Job drawing, mm, ordinate dimensions from the low corner. One solid piece. A direction names the side the tool comes from. Coordinates: 2 decimals unless noted, no trailing zeros. Order: outer loops, then holes, each group sorted by start corner. A loop starts at its lowest first (then second) coordinate and runs counter-clockwise, first axis right, second up. Notation, with made-up numbers: (-34.5, -22) - (-13.5, -22) arc R7 ccw to (-13.5, -17) - close; hole circle Ø9 at (44, 32). An arc over 180 degrees is marked (long way). Use one line per item in the form item = value.
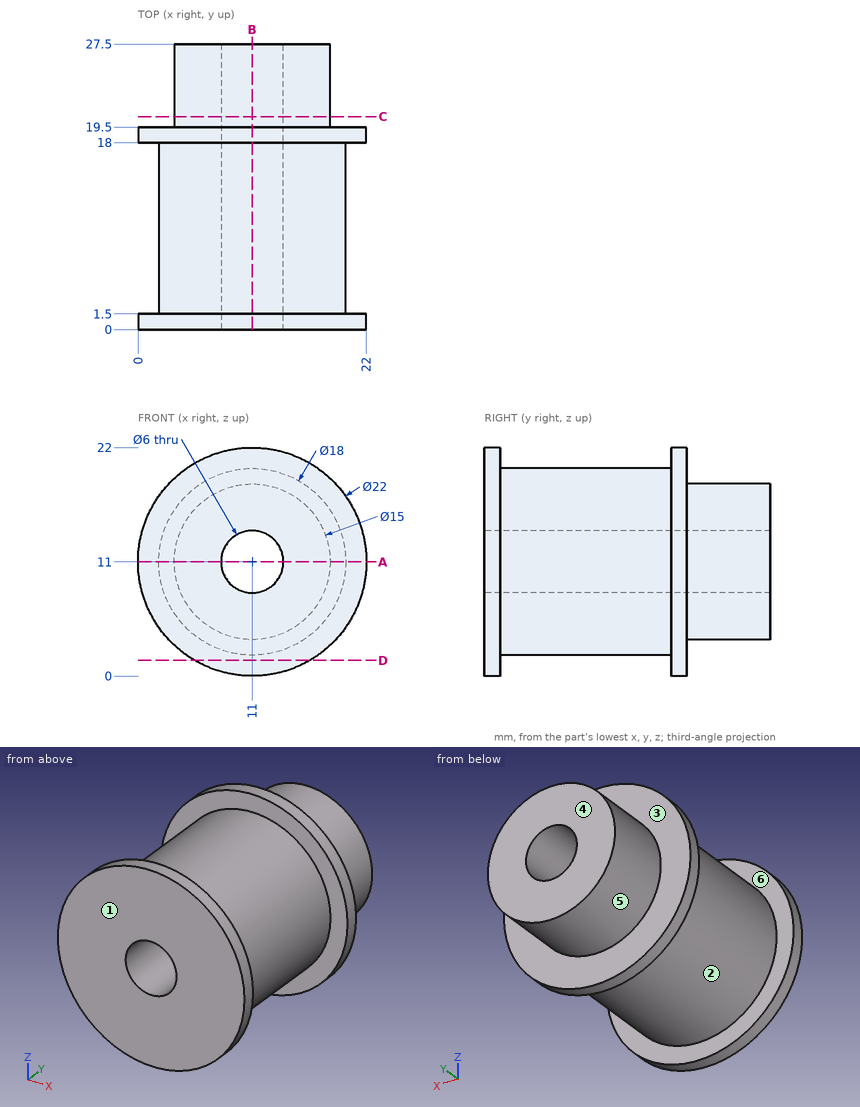
Item 1: Cut at B-B, the plane x = 11. Write the cut outline in (y, z), plus the area to 3 significant figures.
Derived:
outline = (0, 0) - (1.5, 0) - (1.5, 2) - (18, 2) - (18, 0) - (19.5, 0) - (19.5, 3.5) - (27.5, 3.5) - (27.5, 8) - (0, 8) - close; (0, 14) - (27.5, 14) - (27.5, 18.5) - (19.5, 18.5) - (19.5, 22) - (18, 22) - (18, 20) - (1.5, 20) - (1.5, 22) - (0, 22) - close
area = 318 mm²
Item 2: Cut at A-A, the plane z = 11. Write the cut outline in (x, y), plus the area to 3 significant figures.
Derived:
outline = (0, 0) - (8, 0) - (8, 27.5) - (3.5, 27.5) - (3.5, 19.5) - (0, 19.5) - (0, 18) - (2, 18) - (2, 1.5) - (0, 1.5) - close; (14, 0) - (22, 0) - (22, 1.5) - (20, 1.5) - (20, 18) - (22, 18) - (22, 19.5) - (18.5, 19.5) - (18.5, 27.5) - (14, 27.5) - close
area = 318 mm²
Item 3: 3-axis set-ups, long thin cutter, end or side, ignore diameter. For the marked faces 1, 2 and 3: which of +Z, -Z, +X, -X, +Y, -Y reach the whole face in a straight line?
Derived:
face_1 = +Z, -Z, +X, -X, -Y
face_2 = none
face_3 = +Y
Item 4: Cut at D-D, the plane z = 1.5. Write the cut outline in (x, y).
Derived:
outline = (5.45, 0) - (16.55, 0) - (16.55, 1.5) - (5.45, 1.5) - close; (5.45, 18) - (16.55, 18) - (16.55, 19.5) - (5.45, 19.5) - close
Item 5: Two-plate mould, pull along Y, no slides. Class the marked faces 4, 5 and 6: +Y half, -Y half, draft (parallel to the pull), parting line (faces both ways), or undercut.
Derived:
face_4 = +Y half
face_5 = draft
face_6 = undercut
Item 6: Drop flat-ended pins along their axis: pin 1 (3 mm diameter, centred on y = 19.5, z = 15.5, fed in from -X); pin 2 (1 mm diameter, centred on y = 3.5, z = 5.5, fed in from +X); pin 3 (2 mm diameter, centred on x = 10, y = 5.5, fed in from -Z). Give the stop position or say it passes through.
Derived:
pin_1 = 0.42
pin_2 = 18.48
pin_3 = 2
Item 7: Drill centre lines: line 1 (Y direction, x = 4, z = 17.5); line 2 (Z direction, x = 11, y = 8.5); line 3 (X direction, y = 12, z = 10.5). Where is each one in solid material? Low to high. Write a range as [from, to].
Derived:
line_1 = [0, 1.5], [18, 19.5]
line_2 = [2, 8], [14, 20]
line_3 = [2.01, 8.04], [13.96, 19.99]
Item 8: Cut at C-C, the plane y = 20.5. Write the cut outline in (x, z), plus the area to 3 significant figures.
Derived:
outline = circle Ø15 at (11, 11); hole circle Ø6 at (11, 11)
area = 148 mm²
